Read the model definition and answer for the solid it produces. Units are mm, in the model's axes. A direction names the side the tool comes from. Coordinates: 2 decimals unless noted, no trailing zeros. Loops run counter-clockwise (first coordinate to the right, second up) from the corner with the lowest first, then second, coordinate; pieces in that order, holes last. Notation, with made-up numbers: M -18.75,-17 L 3.25,-17 A33 ccw 3.25,12 Z; hole C 74,84 d3. An arc over 180 degrees is marked long. One line per item, written item: value. Start each with the question number.
1. The part is cut by section C-C (x = 2.25). Write down the section's boundary in (y, z), then the cut area to 3 significant figures.
2. Determine the mould class of faces 1 (the face through (2, 7.5, 12)), 2 (the face through (0, 2, 14)), 3 (the face through (7.58, -2.44, 13.04)) for opening direction Z: +Z half, -Z half, draft (parallel to the pull), parting line (faces both ways), or undercut.
3. For faces 4 (the face through (12, 5.5, 12)), 5 (the face through (14, 3, 14)), 6 (the face through (0, -2, 25)), determine the directions among +Z, -Z, +X, -X, +Y, -Y from which every point of the face is accessible in a straight line to the end or side of a thin tool.
4. The part is cut by section A-A (x = 0). Write down the section's boundary in (y, z).
5. The part is cut by section D-D (z = 19). Write down the section's boundary in (x, y).
6. The part is cut by section B-B (z = 12.5). Write down the section's boundary in (x, y).
7. Flat-ended cylindrical pins translate along their axes: pin 1 (1.5 mm diameter, centred on x = 12, z = 11.5, fed in from +Y); pin 2 (1 mm diameter, centred on y = -2.5, z = 15, fed in from +X); pin 3 (4 mm diameter, centred on y = -2, z = 16, fed in from +X). Find the tip coordinate at first contact, or state that the pin passes through.
8. Consider probe 1 along X at (y, z) = (4.25, 12.5); probe 2 along Z at (x, y) = (0, -0.25); probe 3 along Z at (x, y) = (0, 4). Determine where each line is inside the solid, lowest interval first.
```python
from build123d import *

# Parameters (mm, degrees)
SKETCH1_R                = 2.5
BOSS_EXTRUDE1_DEPTH      = 12.5
SKETCH2_R                = 1.5
BOSS_EXTRUDE2_DEPTH      = 5
SKETCH4_R                = 2.5
BOSS_EXTRUDE3_DEPTH      = 12.5
SKETCH5_R                = 2.5
BOSS_EXTRUDE4_DEPTH      = 3
SKETCH6_R                = 1.5
BOSS_EXTRUDE5_DEPTH      = 2.5
REVOLVE2_ANGLE           = 90
REVOLVE3_ANGLE           = 90
SKETCH18_R               = 3.75
BOSS_EXTRUDE6_DEPTH      = 7.5
BOSS_EXTRUDE6_DEPTH_BACK = 3.5
SKETCH20_R               = 1.5
CUT_EXTRUDE2_DEPTH       = 1.0000001
CUT_EXTRUDE2_DEPTH_BACK  = 12.0000001
CUT_EXTRUDE3_DEPTH       = 1.0000001
CUT_EXTRUDE3_DEPTH_BACK  = 12.0000001


with BuildPart() as part:
    # Sketch1 → Boss-Extrude1 (new body)
    with BuildSketch(Plane.XY):
        Circle(SKETCH1_R)
    boss_extrude1 = extrude(amount=BOSS_EXTRUDE1_DEPTH)

    # Sketch2 → Boss-Extrude2 (add)
    with BuildSketch(Plane(origin=(0, 0, 0), x_dir=(-1, 0, 0), z_dir=(0, 0, -1))):
        Circle(SKETCH2_R)
    boss_extrude2 = extrude(amount=BOSS_EXTRUDE2_DEPTH)

    # Sketch4 → Boss-Extrude3 (add)
    with BuildSketch(Plane(origin=(0, 0, 0), x_dir=(0, 0, -1), z_dir=(1, 0, 0))):
        with Locations((-12.5, 0)):
            Circle(SKETCH4_R)
    extrude(amount=BOSS_EXTRUDE3_DEPTH)

    # Sketch5 → Boss-Extrude4 (add)
    with BuildSketch(Plane(origin=(0, 0, 0), x_dir=(1, 0, 0), z_dir=(0, 1, 0))):
        with Locations((12.5, -12.5)):
            Circle(SKETCH5_R)
    extrude(amount=BOSS_EXTRUDE4_DEPTH)

    # Sketch6 → Boss-Extrude5 (add)
    with BuildSketch(Plane(origin=(0, 3, 0), x_dir=(1, 0, 0), z_dir=(0, 1, 0))):
        with Locations((12.5, -12.5)):
            Circle(SKETCH6_R)
    extrude(amount=BOSS_EXTRUDE5_DEPTH)

    # Sketch8 → Revolve2 (revolve)
    with BuildSketch(Plane.ZY):
        with BuildLine():
            Line((12.5, 2.5), (12.5, -2.5))
            ThreePointArc((12.5, -2.5), (15, 0), (12.5, 2.5))
        make_face()
    revolve(axis=Axis((0, 2.5, 12.5), (0, -1, 0)), revolution_arc=REVOLVE2_ANGLE)

    # Sketch16 → Revolve3 (revolve)
    with BuildSketch(Plane.XZ):
        with BuildLine():
            Line((12.5, 15), (12.5, 10))
            ThreePointArc((12.5, 10), (15, 12.5), (12.5, 15))
        make_face()
    revolve(axis=Axis((12.5, 0, 15), (0, 0, -1)), revolution_arc=REVOLVE3_ANGLE)

    # Sketch18 → Boss-Extrude6 (add, two sides)
    with BuildSketch(Plane(origin=(0, 0, 0), x_dir=(1, 0, 0), z_dir=(0, 1, 0))) as boss_extrude6_sk:
        with Locations((0, -12.5)):
            Circle(SKETCH18_R)
    extrude(amount=BOSS_EXTRUDE6_DEPTH)
    extrude(boss_extrude6_sk.sketch, amount=-BOSS_EXTRUDE6_DEPTH_BACK)

    # Mirror1: Boss-Extrude1, Boss-Extrude2 across plane
    add(boss_extrude1.mirror(Plane.XY.offset(12.5)))
    add(boss_extrude2.mirror(Plane.XY.offset(12.5)))

    # Sketch20 → Cut-Extrude2 (cut, two sides)
    with BuildSketch(Plane(origin=(0, 7.5, 0), x_dir=(1, 0, 0), z_dir=(0, 1, 0))) as cut_extrude2_sk:
        with Locations((0, -12.5)):
            Circle(SKETCH20_R)
    extrude(amount=CUT_EXTRUDE2_DEPTH, mode=Mode.SUBTRACT)
    extrude(cut_extrude2_sk.sketch, amount=-CUT_EXTRUDE2_DEPTH_BACK, mode=Mode.SUBTRACT)

    # Sketch21 → Cut-Extrude3 (cut, two sides)
    with BuildSketch(Plane(origin=(0, 7.5, 0), x_dir=(1, 0, 0), z_dir=(0, 1, 0))) as cut_extrude3_sk:
        with BuildLine():
            Line((2.653299832, -9.85), (12.281852951, 10.075018896))
            Line((12.281852951, 10.075018896), (-12.7945827, 9.436331987))
            Line((-12.7945827, 9.436331987), (-2.653299832, -9.85))
            ThreePointArc((-2.653299832, -9.85), (0, -8.75), (2.653299832, -9.85))
        make_face()
    extrude(amount=CUT_EXTRUDE3_DEPTH, mode=Mode.SUBTRACT)
    extrude(cut_extrude3_sk.sketch, amount=-CUT_EXTRUDE3_DEPTH_BACK, mode=Mode.SUBTRACT)


solid = part.part
```
Answer block:
1. outline: M -3.5,9.5 L 7.5,9.5 L 7.5,15.5 L 1.09,15.5 L 1.09,25 L -1.09,25 L -1.09,15.5 L -3.5,15.5 Z
1. area: 86.7 mm2
2. face 1: draft
2. face 2: undercut
2. face 3: parting line
3. face 4: +Z, -Z, +X, +Y
3. face 5: +Y
3. face 6: +Z
4. outline: M -3.5,8.75 L 7.5,8.75 L 7.5,11 L -3.5,11 Z; M -3.5,14 L 7.5,14 L 7.5,16.25 L 2.5,16.25 L 2.5,25 L 1.5,25 L 1.5,30 L -1.5,30 L -1.5,25 L -2.5,25 L -2.5,16.25 L -3.5,16.25 Z
5. outline: C 0,0 d5
6. outline: M -3.75,-3.5 L -1.5,-3.5 L -1.5,7.5 L -3.75,7.5 Z; M 1.5,-3.5 L 3.75,-3.5 L 3.75,-2.5 L 12.5,-2.5 A2.5 ccw 15,0 L 15,3 L 14,3 L 14,5.5 L 11,5.5 L 11,3 L 10,3 L 10,2.5 L 3.75,2.5 L 3.75,7.5 L 1.5,7.5 Z
7. pin 1: stops at y = 5.5
7. pin 2: stops at x = 3.17
7. pin 3: stops at x = 13.96
8. probe 1: x = -3.75 to -1.5, 1.5 to 3.75, 11 to 14
8. probe 2: z = 8.75 to 11, 14 to 30
8. probe 3: z = 8.75 to 11, 14 to 16.25
